from build123d import *

# Parameters (mm, degrees)
ESQUISSE2_R             = 150
BOSS_EXTRU_1_DEPTH      = 150
ESQUISSE3_R             = 148
ENL_V_MAT_EXTRU_1_DEPTH = 148
ESQUISSE5_R             = 150
BOSS_EXTRU_2_DEPTH      = 150
ESQUISSE6_R             = 148
ENL_V_MAT_EXTRU_2_DEPTH = 177
ESQUISSE7_R             = 148
BOSS_EXTRU_3_DEPTH      = 2
ESQUISSE9_R             = 20
ENL_V_MAT_EXTRU_3_DEPTH = 200


with BuildPart() as part:
    # Esquisse2 → Boss.-Extru.1 (new body)
    with BuildSketch(Plane(origin=(0, 0, 0), x_dir=(1, 0, 0), z_dir=(0, 1, 0))):
        Circle(ESQUISSE2_R)
    extrude(amount=BOSS_EXTRU_1_DEPTH)

    # Esquisse3 → Enlèv. mat.-Extru.1 (cut)
    with BuildSketch(Plane(origin=(0, 0, 0), x_dir=(1, 0, 0), z_dir=(0, 1, 0))):
        Circle(ESQUISSE3_R)
    extrude(amount=ENL_V_MAT_EXTRU_1_DEPTH, mode=Mode.SUBTRACT)

    # Esquisse5 → Boss.-Extru.2 (add)
    with BuildSketch(Plane(origin=(0, 150, 0), x_dir=(1, 0, 0), z_dir=(0, 1, 0))):
        with Locations((0, -2)):
            Circle(ESQUISSE5_R)
    extrude(amount=-BOSS_EXTRU_2_DEPTH)

    # Esquisse6 → Enlèv. mat.-Extru.2 (cut)
    with BuildSketch(Plane(origin=(0, 0, 0), x_dir=(1, 0, 0), z_dir=(0, 1, 0))):
        Circle(ESQUISSE6_R)
    extrude(amount=ENL_V_MAT_EXTRU_2_DEPTH, mode=Mode.SUBTRACT)

    # Esquisse7 → Boss.-Extru.3 (add)
    with BuildSketch(Plane.XZ):
        Circle(ESQUISSE7_R)
    extrude(amount=-BOSS_EXTRU_3_DEPTH)

    # Esquisse9 → Enlèv. mat.-Extru.3 (cut)
    with BuildSketch(Plane.XY):
        with Locations((-100, 76)):
            Circle(ESQUISSE9_R)
        with Locations((100, 76)):
            Circle(ESQUISSE9_R)
    extrude(amount=ENL_V_MAT_EXTRU_3_DEPTH, mode=Mode.SUBTRACT)


solid = part.part
The listing builds one solid part. Answer for the finished solid, in the listing's coordinates (mm). A direction names the side the tool comes from. Round coordinates to 2 decimals unless told otherwise and drop trailing zeros. Write each loop counter-clockwise with the first axis right and the second up, starting at its lowest first coordinate (ties: lowest second). Pieces come first, ordered by that corner, then holes. Notation, with made-up numbers: M 56.5,34 L 66.5,34 A19 cw 66.5,49 Z; hole C 36.25,45 d4. An arc over 180 degrees is marked long. Write each question's results on one line, items separated by ' | '. Start each with the question number.
Item 1: Flat-ended cylindrical pins translate along their axes: pin 1 Ø12 at (x, z) = (-30.5, -42.5) entering from +Y; pin 2 Ø5 at (x, y) = (-63, 51.5) entering from -Z; pin 3 Ø1.5 at (x, y) = (-65, 75) entering from -Z. Find the tip coordinate at first contact, or state that the pin passes through.
Item 2: A cutting plane is placed at B-B on z = 104.5. Write down the section's boundary in (x, y).
Item 3: For faces 1 (the face through (33, 150, 146)), 2 (the face through (-2, 2, 2)), 3 (the face through (-103.761, 56.357, 109.222)), determine the directions among +Z, -Z, +X, -X, +Y, -Y from which every point of the face is accessible in a straight line to the end or side of a thin tool.
Item 4: A cutting plane is placed at D-D on x = 43. Write down the section's boundary in (y, z).
Item 5: For a pull along X with two mould halves and no side action, classify faces 4 (the face through (105.455, 56.758, 107.657)), 5 (the face through (3.312, 73.95, -149.963)), 6 (the face through (-2, 0, 3)) as pulls with the +X half, pulls with the -X half, needs draft (parallel to the pull), parting line crosses it, or undercut.
Item 6: Straight lines are drawn through the part: L1, parallel to Y at x = 100, z = 112.5; L2, parallel to Y at x = 39, z = 36; L3, parallel to X at y = 54, z = 106.5. For each, find the intervals that lie inside material, in ascending order. Write a range as [from, to].
Item 7: A cutting plane is placed at C-C on x = -93.5. Write down the section's boundary in (y, z).
Check sheet entries:
1) pin 1: y = 2 | pin 2: z = -137.26 | pin 3: z = -135.54
2) outline: M -109.52,0 L 109.52,0 L 109.52,58.41 A20 cw 104.8,56.59 L 104.8,2 L -104.8,2 L -104.8,56.59 A20 cw -109.52,58.41 Z; M -109.52,93.59 A20 cw -104.8,95.41 L -104.8,150 L -109.52,150 Z; M 104.8,95.41 A20 cw 109.52,93.59 L 109.52,150 L 104.8,150 Z
3) face 1: +Z, -Z, +X, -X, +Y | face 2: +Y | face 3: +Z
4) outline: M 0,-143.7 L 150,-143.7 L 150,-141.62 L 2,-141.62 L 2,141.62 L 150,141.62 L 150,145.7 L 0,145.7 Z
5) face 4: undercut | face 5: parting line crosses it | face 6: needs draft
6) L1: [0, 56], [96, 150] | L2: [0, 2] | L3: [-107.61, -102.77], [102.77, 107.61]
7) outline: M 0,-117.29 L 150,-117.29 L 150,-114.72 L 2,-114.72 L 2,114.72 L 57.09,114.72 L 57.09,119.29 L 0,119.29 Z; M 94.91,114.72 L 150,114.72 L 150,119.29 L 94.91,119.29 Z
